Read the model definition and answer for the solid it produces. Units are mm, in the model's axes. Face numbers are marked on the shaded views. A direction names the side the tool comes from. Coordinates: 2 decimals unless noted, no trailing zeros. Write each loop counter-clockwise with the first axis right and the second up, starting at its lowest first coordinate (ties: lowest second). Pieces come first, ordered by that corner, then holes.
Item 1: A tool of negligible diameter and unlimited length cuts with its end or side. For the marked faces 4, 5 and 6, from which of +Z, -Z, +X, -X, +Y, -Y can it reach the whole face along a straight path? Write none if from no direction.
Item 2: Each of these flat-tipped pins is pushed along its axis until it touches: P1, Ø2, axis at x = -37.5, y = -40.5, coming from the +Z side; P2, Ø6, axis at x = -3.5, z = -13, coming from the -Y side; P3, Ø8, axis at x = 37.5, y = -43.5, coming from the -Z side; P4, Ø12, axis at x = -26, z = 28, coming from the +Y side. Where does it stop, or does it pass through?
Item 3: Straight lines are drawn through the part: probe 1 along Z at (x, y) = (32, -11); probe 2 along Z at (x, y) = (27, 4.5); probe 3 along Y at (x, z) = (0, -76). For each, find the intervals that lie inside material, in ascending order.
Item 4: Section C-C (y = 0) is taken. Give the vertices of the cut face in (x, z), then the cut area to 3 significant figures.
Item 5: Determine the mould class of the marked faces 1, 2 and 3 for opening direction Z: released by +Z, released by -Z, zero draft, split by the parting line, or undercut.
Item 6: Section B-B (x = 36) is taken. Give the vertices of the cut face in (y, z), then the cut area to 3 significant figures.
Item 7: Section A-A (y = -39.5) is taken. Give the vertices of the cut face in (x, z).
from build123d import *


with BuildPart() as part:
    # Esquisse1 → R_volution1 (revolve)
    with BuildSketch(Plane(origin=(0, 0, 0), x_dir=(1, 0, 0), z_dir=(0, 1, 0)), mode=Mode.PRIVATE) as r_volution1_sk:
        Polygon((0, 100), (-27.5, 100), (-27.5, 50), (-42.5, 50), (-42.5, 0), (-25, 0), (-25, -50), (-55, -50), (-55, -100), (0, -100), align=None)
    revolve(r_volution1_sk.sketch.rotate(Axis((0, 0, 100), (0, 0, -1)), 180), axis=Axis((0, 0, 100), (0, 0, -1)))  # turned: the seam where the file's is


solid = part.part
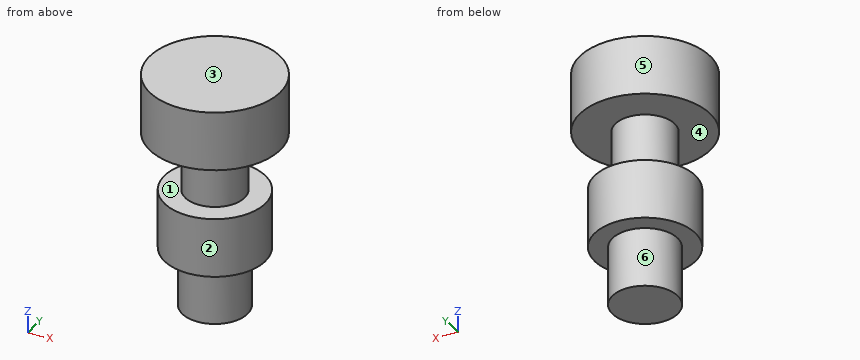
Established:
1. face 4: none
1. face 5: +Z, -Z
1. face 6: -Z
2. P1: stops at z = 100
2. P2: stops at y = -42.5
2. P3: stops at z = 50
2. P4: stops at y = 15
3. probe 1: z = -50 to 0, 50 to 100
3. probe 2: z = -100 to 0, 50 to 100
3. probe 3: y = -27.5 to 27.5
4. outline: (-55, 50) - (-25, 50) - (-25, 0) - (-42.5, 0) - (-42.5, -50) - (-27.5, -50) - (-27.5, -100) - (27.5, -100) - (27.5, -50) - (42.5, -50) - (42.5, 0) - (25, 0) - (25, 50) - (55, 50) - (55, 100) - (-55, 100) - close
4. area: 15,000 mm2
5. face 1: undercut
5. face 2: zero draft
5. face 3: released by +Z
6. outline: (-41.58, 50) - (41.58, 50) - (41.58, 100) - (-41.58, 100) - close; (-22.59, -50) - (22.59, -50) - (22.59, 0) - (-22.59, 0) - close
6. area: 6,420 mm2
7. outline: (-38.27, 50) - (38.27, 50) - (38.27, 100) - (-38.27, 100) - close; (-15.68, -50) - (15.68, -50) - (15.68, 0) - (-15.68, 0) - close
